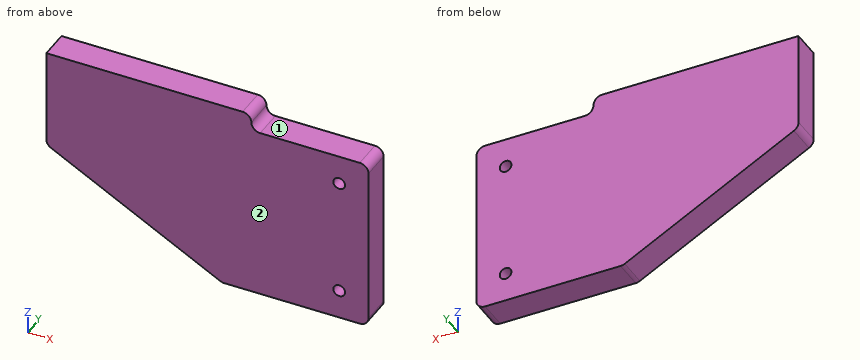
from build123d import *

# Parameters (mm, degrees)
SKETCH1_R           = 1.27
BOSS_EXTRUDE1_DEPTH = 6.4008


with BuildPart() as part:
    # Sketch1 → Boss-Extrude1 (new body)
    with BuildSketch(Plane(origin=(0, 0, 0), x_dir=(1, 0, 0), z_dir=(0, 1, 0))):
        with BuildLine():
            Line((1.905, 0), (23.495, 0))
            ThreePointArc((23.495, 0), (24.842038418, 0.557961582), (25.4, 1.905))
            Line((25.4, 1.905), (25.4, 36.195))
            ThreePointArc((25.4, 36.195), (24.842038418, 37.542038418), (23.495, 38.1))
            Line((23.495, 38.1), (-5.87375, 38.1))
            ThreePointArc((-5.87375, 38.1), (-6.335780366, 38.043121463), (-6.770220588, 37.875882353))
            Line((-6.770220588, 37.875882353), (-43.441470588, 18.317882353))
            ThreePointArc((-43.441470588, 18.317882353), (-44.178524023, 17.617114414), (-44.45, 16.637))
            Line((-44.45, 16.637), (-44.45, -3.81))
            Line((-44.45, -3.81), (-1.905, -3.81))
            ThreePointArc((-1.905, -3.81), (-0.557961582, -3.252038418), (0, -1.905))
            ThreePointArc((0, -1.905), (0.557961582, -0.557961582), (1.905, 0))
        make_face()
        with Locations(Location((19.05, 31.75, 0), (0, 0, 270))):
            Circle(SKETCH1_R, mode=Mode.SUBTRACT)
        with Locations(Location((19.05, 6.35, 0), (0, 0, 270))):
            Circle(SKETCH1_R, mode=Mode.SUBTRACT)
    extrude(amount=BOSS_EXTRUDE1_DEPTH)


solid = part.part
The listing builds one solid part. Answer for the finished solid, in the listing's coordinates (mm). Face numbers are marked on the shaded views. A direction names the side the tool comes from. Give positions to 0.01 mm unless a question says otherwise; leave off trailing zeros. Loops run counter-clockwise (first coordinate to the right, second up) from the corner with the lowest first, then second, coordinate; pieces in that order, holes last.
Item 1: A cutting plane is placed at C-C (z = -6.35). Give the vertices of the cut face in (x, y).
Derived:
outline: (-44.45, 0) - (17.78, 0) - (17.78, 6.4) - (-44.45, 6.4) - close; (20.32, 0) - (25.4, 0) - (25.4, 6.4) - (20.32, 6.4) - close
Item 2: A cutting plane is placed at D-D (z = -31.75). Give the vertices of the cut face in (x, y), then the cut area to 3 significant figures.
Derived:
outline: (-18.26, 0) - (17.78, 0) - (17.78, 6.4) - (-18.26, 6.4) - close; (20.32, 0) - (25.4, 0) - (25.4, 6.4) - (20.32, 6.4) - close
area: 263 mm2
Item 3: Each of these flat-tipped pins is pushed along its axis until it touches: pin 1 Ø12 at (x, z) = (4.5, -26.5) entering from -Y; pin 2 Ø1.9 at (x, y) = (14, 4.5) entering from +Z; pin 3 Ø1.5 at (x, z) = (19.05, -31.75) entering from +Y. Where does it stop, or does it pass through?
Derived:
pin 1: stops at y = 0
pin 2: stops at z = 0
pin 3: passes through
Item 4: A tool of negligible diameter and unlimited length cuts with its end or side. For the marked faces 1 and 2, from which of +Z, -Z, +X, -X, +Y, -Y can it reach the whole face along a straight path? Write none if from no direction.
Derived:
face 1: +Z, +X, +Y, -Y
face 2: +Z, -Z, +X, -X, -Y
Item 5: Find the intervals of material crossed by line 1 along X through (y, z) = (4.25, -6.35); line 2 along Z through (x, y) = (-6, 4.75); line 3 along X through (y, z) = (3.5, 2), in increasing order.
Derived:
line 1: x = -44.45 to 17.78, 20.32 to 25.4
line 2: z = -38.1 to 3.81
line 3: x = -44.45 to 0
Item 6: A cutting plane is placed at A-A (x = 19.05). Give the vertices of the cut face in (y, z), then the cut area to 3 significant figures.
Derived:
outline: (0, -38.1) - (6.4, -38.1) - (6.4, -33.02) - (0, -33.02) - close; (0, -30.48) - (6.4, -30.48) - (6.4, -7.62) - (0, -7.62) - close; (0, -5.08) - (6.4, -5.08) - (6.4, 0) - (0, 0) - close
area: 211 mm2
Item 7: A cutting plane is placed at B-B (y = 4). Give the vertices of the cut face in (x, z) (3 decimals).
Derived:
outline: (-44.45, -16.637) arc R1.905 ccw to (-43.441, -18.318) - (-6.77, -37.876) arc R1.905 ccw to (-5.874, -38.1) - (23.495, -38.1) arc R1.905 ccw to (25.4, -36.195) - (25.4, -1.905) arc R1.905 ccw to (23.495, 0) - (1.905, 0) arc R1.905 cw to (0, 1.905) arc R1.905 ccw to (-1.905, 3.81) - (-44.45, 3.81) - close; hole circle Ø2.54 at (19.05, -31.75); hole circle Ø2.54 at (19.05, -6.35)
